```python
from build123d import *

# Parameters (mm, degrees)
F0_R     = 26.625
F1_DEPTH = 20
F2_SIZE  = 1.5


with BuildPart() as f1:
    # F0 (on Top) → F1 (new body)
    with BuildSketch(Plane.XY):
        with BuildLine():
            ThreePointArc((0, 2), (0.585786, 0.585786), (2, 0))
            Line((2, 0), (7, 0))
            ThreePointArc((7, 0), (9.12132, 0.87868), (10, 3))
            Line((10, 3), (10, 45.4))
            ThreePointArc((10, 45.4), (7.071068, 52.471068), (0, 55.4))
            Line((0, 55.4), (-85.179761, 55.4))
            ThreePointArc((-85.179761, 55.4), (-92.497433, 57.306044), (-97.955397, 62.539776))
            ThreePointArc((-97.955397, 62.539776), (-167.944402, 42.081483), (-97.292796, 24.043935))
            ThreePointArc((-97.292796, 24.043935), (-91.796155, 29.594114), (-84.254223, 31.628032))
            Line((-84.254223, 31.628032), (-26.3, 31.628032))
            ThreePointArc((-26.3, 31.628032), (-19.228932, 28.6991), (-16.3, 21.628032))
            Line((-16.3, 21.628032), (-16.3, 3))
            ThreePointArc((-16.3, 3), (-15.42132, 0.87868), (-13.3, 0))
            Line((-13.3, 0), (-8.3, 0))
            ThreePointArc((-8.3, 0), (-6.885786, 0.585786), (-6.3, 2))
            Line((-6.3, 2), (-6.3, 30))
            Line((-6.3, 30), (0, 30))
            Line((0, 30), (0, 2))
        make_face()
        with Locations((-130.15, 42.73201)):
            Circle(F0_R, mode=Mode.SUBTRACT)
    extrude(amount=F1_DEPTH)

    # F2
    f2_edges = [f1.edges().sort_by_distance(p)[0] for p in [
        (-156.775, 42.73201, 0),
        (-156.775, 42.73201, 20),
    ]]
    chamfer(f2_edges, length=F2_SIZE)


solid = f1.part
```
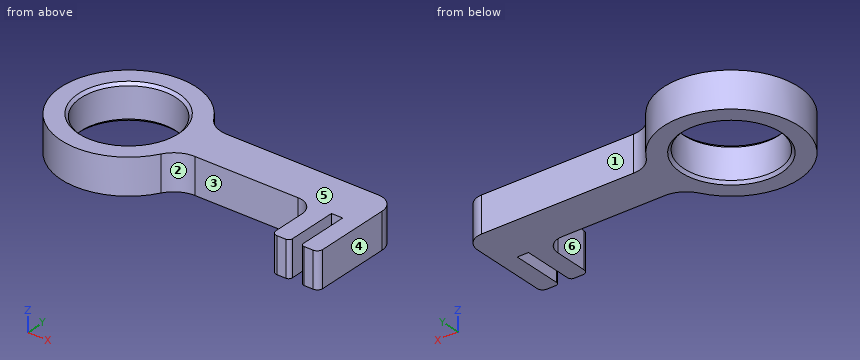
Check sheet for the modelled part. Datum: model origin and axes. Units: mm. Face numbers are marked on the shaded views. A direction names the side the tool comes from. Round coordinates to 2 decimals unless told otherwise and drop trailing zeros. Order: outer loops, then holes, each group sorted by start corner. A loop starts at its lowest first (then second) coordinate and runs counter-clockwise, first axis right, second up.
1) Go/stop test with flat-tipped pins: pin 1 Ø9.5 at (y, z) = (12, 7) entering from -X; pin 2 Ø8 at (x, z) = (-82.5, 3.5) entering from +Y; pin 3 Ø12 at (x, y) = (-25.5, 14) entering from -Z; pin 4 Ø10 at (x, z) = (-58.5, 5) entering from -Y. Record where each tip stops, or that it passes through.
2) Section check B-B (z = 5). Record the boundary of the cut face in (x, y) (3 decimals), and give its area (3 significant figures).
3) Mould release check, pull along X, two halves, no side actions. Record for the marked faces 1, 2, 3 and 4: +X half, -X half, draft (parallel to the pull), parting line (faces both ways), or undercut.
4) Section check A-A (x = -130.15). Record the boundary of the cut face in (y, z).
5) Tool access check on the marked faces 5 and 6. Record the directions out of +Z, -Z, +X, -X, +Y, -Y that give a thin tool (end or side, any length) a straight path to the whole face; none if there is none.
6) Section check D-D (x = -10). Record the boundary of the cut face in (y, z).
7) Section check C-C (y = 27.5). Give the number of separate pieces and of enclosed holes in the cut face, and give its area (3 significant figures).
8) Scan lines: line 1 (X direction, y = 43, z = 14.25); line 2 (X direction, y = 25.5, z = 7); line 3 (Y direction, x = -130.15, z = 9). Record each from-to range of solid material in increasing order.
Result:
1. pin 1: stops at x = -157.6
1. pin 2: stops at y = 55.46
1. pin 3: passes through
1. pin 4: stops at y = 31.63
2. outline: (-97.955, 62.54) arc R37.8 ccw (long way) to (-97.293, 24.044) arc R15 cw to (-84.254, 31.628) - (-26.3, 31.628) arc R10 cw to (-16.3, 21.628) - (-16.3, 3) arc R3 ccw to (-13.3, 0) - (-8.3, 0) arc R2 ccw to (-6.3, 2) - (-6.3, 30) - (0, 30) - (0, 2) arc R2 ccw to (2, 0) - (7, 0) arc R3 ccw to (10, 3) - (10, 45.4) arc R10 ccw to (0, 55.4) - (-85.18, 55.4) arc R15 cw to start; hole circle Ø53.25 at (-130.15, 42.732)
2. area: 5,380 mm2
3. face 1: draft
3. face 2: undercut
3. face 3: undercut
3. face 4: +X half
4. outline: (4.93, 0) - (14.61, 0) - (16.11, 1.5) - (16.11, 18.5) - (14.61, 20) - (4.93, 20) - close; (69.36, 1.5) - (70.86, 0) - (80.53, 0) - (80.53, 20) - (70.86, 20) - (69.36, 18.5) - close
5. face 5: +Z, +X, -X, +Y, -Y
5. face 6: +Z, -Z, -Y
6. outline: (0, 0) - (55.4, 0) - (55.4, 20) - (0, 20) - close
7. separate pieces: 4
7. enclosed holes: 0
7. area: 962 mm2
8. line 1: x = -167.95 to -156.77, -103.53 to 10
8. line 2: x = -163.79 to -150.45, -109.85 to -96.35, -17.08 to -6.3, 0 to 10
8. line 3: y = 4.93 to 16.11, 69.36 to 80.53
